Read the model definition and answer for the solid it produces. Units are mm, in the model's axes. Coordinates: 2 decimals unless noted, no trailing zeros. Write each loop counter-clockwise with the first axis right and the second up, starting at its lowest first coordinate (ties: lowest second). Pieces come first, ordered by that corner, then holes. Notation, with made-up numbers: (25, 43.5) - (39, 43.5) arc R15 cw to (39, 70.5) - close; hole circle Ø6 at (70, 57). An arc over 180 degrees is marked (long way). Return JSON: item names as keys, results as strings.
```python
from build123d import *

# Parameters (mm, degrees)
SKETCH1_R           = 7
SKETCH1_R_2         = 4.5
BOSS_EXTRUDE1_DEPTH = 2
CHAMFER1_SIZE       = 1
CHAMFER2_SIZE       = 0.5


with BuildPart() as part:
    # Sketch1 → Boss-Extrude1 (new body)
    with BuildSketch(Plane(origin=(0, 0, 0), x_dir=(1, 0, 0), z_dir=(0, 1, 0))):
        Circle(SKETCH1_R)
        Circle(SKETCH1_R_2, mode=Mode.SUBTRACT)
    extrude(amount=BOSS_EXTRUDE1_DEPTH)

    # Chamfer1
    chamfer1_edges = [part.edges().sort_by_distance(p)[0] for p in [
        (-7, 2, 0),
    ]]
    chamfer(chamfer1_edges, length=CHAMFER1_SIZE)

    # Chamfer2
    chamfer2_edges = [part.edges().sort_by_distance(p)[0] for p in [
        (-7, 0, 0),
        (-4.5, 0, 0),
        (-4.5, 2, 0),
    ]]
    chamfer(chamfer2_edges, length=CHAMFER2_SIZE)


solid = part.part
```
(1) A cutting plane is placed at C-C (y = 0.2). Determine the outline of the cut face in (x, z), and give its area (3 significant figures).
Answer:
{"outline": "circle Ø13.4 at (0, 0); hole circle Ø9.6 at (0, 0)", "area": "68.6 mm²"}
(2) Determine the mould class of faces 1 (the face through (-4, 2, -4)), 2 (the face through (6.466, 0.746, 2.681)), 3 (the face through (-0.59, 0.99, -4.46)) for opening direction X: +X half, -X half, draft (parallel to the pull), parting line (faces both ways), or undercut.
Answer:
{"face 1": "draft", "face 2": "parting line", "face 3": "undercut"}
(3) A cutting plane is placed at A-A (z = 0). Determine the outline of the cut face in (x, y).
Answer:
{"outline": "(-7, 0.5) - (-6.5, 0) - (-5, 0) - (-4.5, 0.5) - (-4.5, 1.5) - (-5, 2) - (-6, 2) - (-7, 1) - close; (4.5, 0.5) - (5, 0) - (6.5, 0) - (7, 0.5) - (7, 1) - (6, 2) - (5, 2) - (4.5, 1.5) - close"}
(4) A cutting plane is placed at B-B (x = 0). Determine the outline of the cut face in (y, z), and give its area (3 significant figures).
Answer:
{"outline": "(0, -6.5) - (0.5, -7) - (1, -7) - (2, -6) - (2, -5) - (1.5, -4.5) - (0.5, -4.5) - (0, -5) - close; (0, 5) - (0.5, 4.5) - (1.5, 4.5) - (2, 5) - (2, 6) - (1, 7) - (0.5, 7) - (0, 6.5) - close", "area": "8.25 mm²"}
(5) Straight lines are drawn through the part: line 1 (X direction, y = 0.8, z = 0); line 2 (Z direction, x = 0, y = 1.1). For each, find the intervals that lie inside material, in ascending order. Write a range as from..to.
Answer:
{"line 1": "-7..-4.5, 4.5..7", "line 2": "-6.9..-4.5, 4.5..6.9"}
